Work out the finished part from the listing and answer in its coordinate system (mm). A direction names the side the tool comes from. Give positions to 0.01 mm unless a question says otherwise; leave off trailing zeros. Order: outer loops, then holes, each group sorted by start corner. A loop starts at its lowest first (then second) coordinate and runs counter-clockwise, first axis right, second up. Notation, with made-up numbers: M 27,36.5 L 33,36.5 A16 cw 33,66.5 Z; hole C 68,78 d1. An arc over 180 degrees is marked long. One line per item, written item: value.
from build123d import *

# Parameters (mm, degrees)
EXTRUDE_1_DEPTH     = 3
EXTRUDE_START       = 3
SKETCH_1_6_R        = 3
EXTRUDE_2_DEPTH     = 15
CUT_EXTRUDE_START   = 18
SKETCH_1_7_R        = 0.65
CUT_EXTRUDE_2_DEPTH = 2
SKETCH_2_R          = 0.75
CUT_EXTRUDE_3_DEPTH = 2


with BuildPart() as part:
    # 草图1 → 凸台-拉伸1 (new body)
    with BuildSketch(Plane.XY):
        with BuildLine():
            Line((-29.444863729, -20), (29.444863729, -20))
            ThreePointArc((29.444863729, -20), (32.04293994, -18.5), (32.04293994, -15.5))
            Line((32.04293994, -15.5), (2.598076211, 35.5))
            ThreePointArc((2.598076211, 35.5), (0, 37), (-2.598076211, 35.5))
            Line((-2.598076211, 35.5), (-32.04293994, -15.5))
            ThreePointArc((-32.04293994, -15.5), (-32.04293994, -18.5), (-29.444863729, -20))
        make_face()
        Polygon((24.248711306, -14), (-24.248711306, -14), (0, 28), align=None, mode=Mode.SUBTRACT)
    extrude(amount=EXTRUDE_1_DEPTH)

    # 草图1<6> → 凸台-拉伸2 (add)
    with BuildSketch(Plane.XY.offset(EXTRUDE_START)):
        with Locations(Location((-29.444863729, -17, 0), (0, 0, 150))):
            Circle(SKETCH_1_6_R)
        with Locations(Location((29.444863729, -17, 0), (0, 0, 270))):
            Circle(SKETCH_1_6_R)
        with Locations(Location((0, 34, 0), (0, 0, 150))):
            Circle(SKETCH_1_6_R)
    extrude(amount=EXTRUDE_2_DEPTH)

    # 草图1<7> → 切除-拉伸2 (cut)
    with BuildSketch(Plane.XY.offset(CUT_EXTRUDE_START)):
        with Locations((0, 34)):
            Circle(SKETCH_1_7_R)
        with Locations((-29.444863729, -17)):
            Circle(SKETCH_1_7_R)
        with Locations((29.444863729, -17)):
            Circle(SKETCH_1_7_R)
    extrude(amount=-CUT_EXTRUDE_2_DEPTH, mode=Mode.SUBTRACT)

    # 草图2 → 切除-拉伸3 (cut)
    with BuildSketch(Plane(origin=(0, 0, 0), x_dir=(-1, 0, 0), z_dir=(0, 0, -1))):
        with Locations((-13.665408814, -17)):
            Circle(SKETCH_2_R)
        with Locations((13.665408814, -17)):
            Circle(SKETCH_2_R)
        with Locations((0, 34)):
            Circle(SKETCH_2_R)
    extrude(amount=-CUT_EXTRUDE_3_DEPTH, mode=Mode.SUBTRACT)


solid = part.part
(1) Find the intervals of material crossed by probe 1 along X at (y, z) = (34, 17.2); probe 2 along Z at (x, y) = (-14.5, -16); probe 3 along Y at (x, z) = (-6.5, 2.25), in increasing order. Write a range as from..to.
Findings:
probe 1: x = -3..-0.65, 0.65..3
probe 2: z = 0..3
probe 3: y = -20..-14, 16.74..28.74
(2) Section C-C, the plane z = 13.5 is taken. Give the vertices of the cut face in (x, y), then the cut area to 3 significant figures.
Findings:
outline: C -29.44,-17 d6; C 0,34 d6; C 29.44,-17 d6
area: 84.8 mm^2
(3) Determine the mould class of faces 5 (the flat face through (-30, -18, 18)), 6 (the cylindrical face through (-14.011, -17.665, 0.986)), 7 (the flat face through (-17.114, 10.357, 1.479)) for opening direction X: pulls with the +X half, pulls with the -X half, needs draft (parallel to the pull), parting line crosses it, or undercut.
Findings:
face 5: needs draft
face 6: undercut
face 7: pulls with the -X half
(4) Section A-A, the plane y = -8 is taken. Give the vertices of the cut face in (x, z), then the cut area to 3 significant figures.
Findings:
outline: M -27.71,0 L -20.78,0 L -20.78,3 L -27.71,3 Z; M 20.78,0 L 27.71,0 L 27.71,3 L 20.78,3 Z
area: 41.6 mm^2
(5) Given P1, Ø5, axis at x = -3, y = 21, coming from the +Z side; P2, Ø1.2, axis at x = 0, y = 34, coming from the -Z side; P3, Ø2.5, axis at x = -7, z = 2, coming from the +Y side, each flat-ended and moving along its own axis, determine where each tip first touches the part or whether it passes through.
Findings:
P1: stops at z = 3
P2: stops at z = 2
P3: stops at y = 30.04
(6) Which of the six approach directions +Z, -Z, +X, -X, +Y, -Y give full straight-line access (tool end or side, diameter ignored) to faces 1 (the flat face through (17.53, 9.64, 1.48)), 2 (the flat face through (-12.29, 6.71, 1.48)), 3 (the flat face through (-14, -17, 2)), 4 (the cylindrical face through (-32.1, -18.4, 10.9))?
Findings:
face 1: +Z, -Z, +X, +Y
face 2: +Z, -Z
face 3: -Z
face 4: +Z
(7) Section B-B, the plane x = 8.5 is taken. Give the vertices of the cut face in (y, z).
Findings:
outline: M -20,0 L -14,0 L -14,3 L -20,3 Z; M 13.28,0 L 25.28,0 L 25.28,3 L 13.28,3 Z
